Check sheet for the drawn part. Datum: minimum x, y, z corner. Units: mm. Give positions to 0.01 mm unless a question says otherwise; leave off trailing zeros. Order: outer loops, then holes, each group sorted by start corner. A loop starts at its lowest first (then second) coordinate and runs counter-clockwise, first axis right, second up.
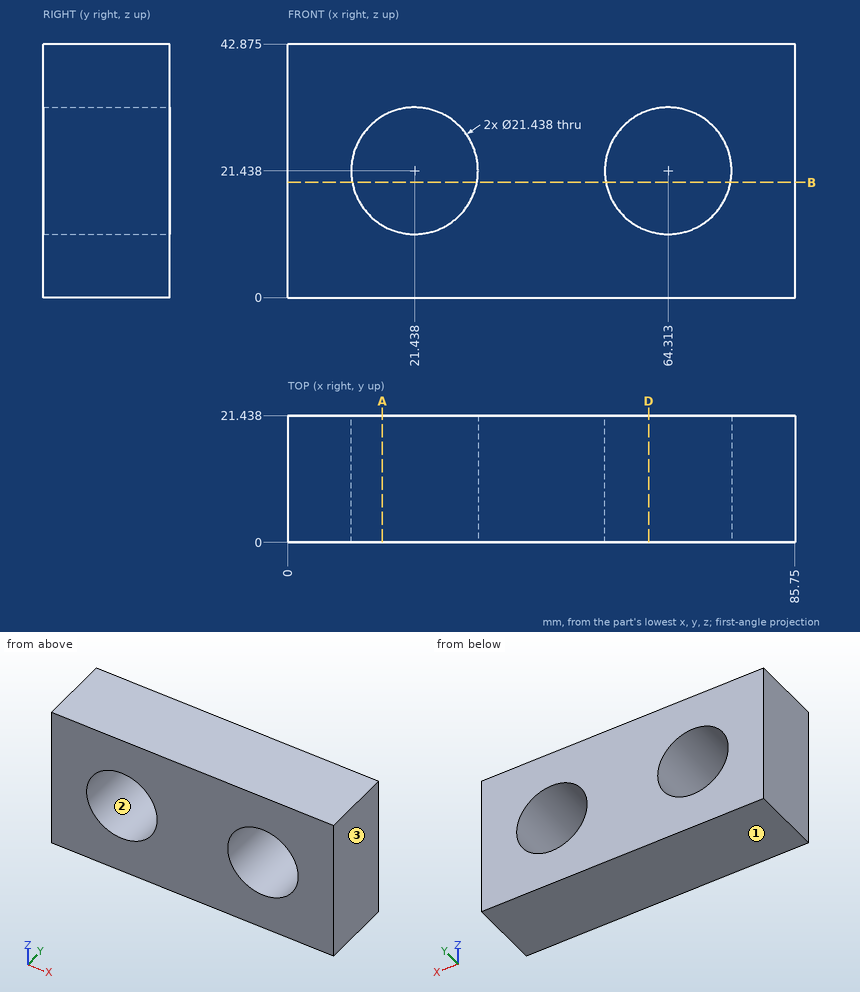
Item 1: Draft check along Z on the marked faces 1, 2 and 3. Enter one of: released by +Z, released by -Z, zero draft, split by the parting line, or undercut.
Reported:
face 1: released by -Z
face 2: undercut
face 3: zero draft
Item 2: Sectioned sample at D-D (x = 61). Enter the section's corners in (y, z) (1 decimal).
Reported:
outline: (0, 0) - (21.4, 0) - (21.4, 11.2) - (0, 11.2) - close; (0, 31.6) - (21.4, 31.6) - (21.4, 42.9) - (0, 42.9) - close
Item 3: Scan lines: L1, parallel to X at y = 1.5, z = 23; L2, parallel to Z at x = 31, y = 11 (1 decimal); L3, parallel to Z at x = 25.5, y = 8.5 (1 decimal). Record each from-to range of solid material in increasing order.
Reported:
L1: x = 0 to 10.83, 32.04 to 53.71, 74.92 to 85.75
L2: z = 0 to 16.6, 26.3 to 42.9
L3: z = 0 to 11.5, 31.4 to 42.9
Item 4: Gauge pin test, flat end, axial feed: pin 1 (17 mm diameter, centred on x = 64.31, z = 21.44, fed in from +Y). Record the tip position at first contact, or that the pin passes through.
Reported:
pin 1: passes through
Item 5: Sectioned sample at A-A (x = 16). Enter the section's corners in (y, z) (1 decimal).
Reported:
outline: (0, 0) - (21.4, 0) - (21.4, 12.2) - (0, 12.2) - close; (0, 30.7) - (21.4, 30.7) - (21.4, 42.9) - (0, 42.9) - close
Item 6: Sectioned sample at B-B (z = 19.5). Give the number of separate pieces and of enclosed holes in the cut face, and give its area (3 significant figures).
Reported:
separate pieces: 3
enclosed holes: 0
area: 934 mm2
